Design review of the part built by this model. Coordinates are the model's own, in mm. A direction names the side the tool comes from. Round coordinates to 2 decimals unless told otherwise and drop trailing zeros. Write each loop counter-clockwise with the first axis right and the second up, starting at its lowest first coordinate (ties: lowest second). Pieces come first, ordered by that corner, then holes. Notation, with made-up numbers: (85, -32.75) -> (102, -32.75) arc R23 ccw to (102, -5.75) -> close; hole circle Ø2 at (16.25, 33). An arc over 180 degrees is marked (long way). Write item = value, one per line. Start each with the question number.
Item 1: Add section C-C, the plane x = 0. State the section outline as (y, z) points (3 decimals), then the cut area to 3 significant figures.
Item 2: Machinability: for faces 1 (the flat face through (6, 0, 0)), 2 (the flat face through (0, 6, -10.833)), 3 (the cylindrical face through (9.067, -14.592, 2.855)), 4 (the flat face through (-6, 0, 0)), 5 (the cylindrical face through (6.948, -6.721, 2.188)), which of the approach directions +Z, -Z, +X, -X, +Y, -Y give a long, thin tool a straight path to every point of the face, cutting with its end or side? Answer none if there is none.
Item 3: Add section B-B, the plane x = -8. State the section outline as (y, z) points (3 decimals).
Item 4: Mouldability with a two-part tool opening along Y and no side actions: class faces 6 (the flat face through (3.203, 6, 0)), 7 (the flat face through (0, -21.031, 0)), 8 (the flat face through (5, -8.331, -6)) as released by +Y, released by -Y, zero draft, split by the parting line, or undercut.
Item 5: To check wall thickness, follow L1, parallel to Y at x = -1.5, z = 8.25; L2, parallel to Y at x = -5, z = -7; L3, parallel to X at y = 10.5, z = -2.25. State the ranges of each line that lie inside material, in increasing order.
Item 6: Add section D-D, the plane y = -16. State the section outline as (x, z) points, then the cut area to 3 significant figures.
Item 7: For pin 1 Ø10 at (y, z) = (-1, 7) entering from -X; pin 2 Ø2.5 at (x, z) = (6.5, 4.5) entering from +Y; pin 3 Ø2 at (y, z) = (-5.5, 8) entering from +X; pin 4 Ø1.5 at (y, z) = (-2, -0.5) entering from -X, all flat-tipped, find the tip position at first contact; note any pin that passes through.
Item 8: Add section A-A, the plane z = 0. State the section outline as (x, y) points (3 decimals), then the cut area to 3 significant figures.
from build123d import *

# Parameters (mm, degrees)
F0_R     = 11.130797
F1_DEPTH = 3.175
F2_W     = 6.405964
F2_H     = 21.666086
F3_DEPTH = 12.7
F4_R     = 9.48328
F5_DEPTH = 5.1562
F6_R     = 7.284162
F7_DEPTH = 8.3312
F8_R     = 9.506324
F9_DEPTH = 12.7


with BuildPart() as f1:
    # F0 (on Front) → F1 (new body)
    with BuildSketch(Plane.XZ):
        Circle(F0_R)
    extrude(amount=F1_DEPTH)

    # F2 (on Front) → F3 (join)
    with BuildSketch(Plane.XZ):
        Rectangle(F2_W, F2_H)
    extrude(amount=-F3_DEPTH)

    # F4 (on Front) → F5 (join)
    with BuildSketch(Plane.XZ):
        Circle(F4_R)
    extrude(amount=F5_DEPTH)

    # F6 (on Front) → F7 (join)
    with BuildSketch(Plane.XZ):
        Circle(F6_R)
    extrude(amount=F7_DEPTH)

    # F8 (on face) → F9 (join)
    with BuildSketch(Plane.XZ.offset(8.3312)):
        Circle(F8_R)
    extrude(amount=F9_DEPTH)


solid = f1.part
Result set:
q1.outline = (-21.031, -9.506) -> (-8.331, -9.506) -> (-8.331, -7.284) -> (-5.156, -7.284) -> (-5.156, -9.483) -> (-3.175, -9.483) -> (-3.175, -11.131) -> (0, -11.131) -> (0, -10.833) -> (12.7, -10.833) -> (12.7, 10.833) -> (0, 10.833) -> (0, 11.131) -> (-3.175, 11.131) -> (-3.175, 9.483) -> (-5.156, 9.483) -> (-5.156, 7.284) -> (-8.331, 7.284) -> (-8.331, 9.506) -> (-21.031, 9.506) -> close
q1.area = 671 mm²
q2.face_1 = +Z, -Z, +X, +Y
q2.face_2 = -Z, +X, -X, +Y
q2.face_3 = -Y
q2.face_4 = +Z, -Z, -X, +Y
q2.face_5 = none
q3.outline = (-21.031, -5.135) -> (-8.331, -5.135) -> (-8.331, 5.135) -> (-21.031, 5.135) -> close; (-5.156, -5.092) -> (-3.175, -5.092) -> (-3.175, -7.739) -> (0, -7.739) -> (0, 7.739) -> (-3.175, 7.739) -> (-3.175, 5.092) -> (-5.156, 5.092) -> close
q4.face_6 = zero draft
q4.face_7 = released by -Y
q4.face_8 = undercut
q5.L1 = -21.03 to -8.33, -5.16 to 12.7
q5.L2 = -21.03 to -8.33, -5.16 to 0
q5.L3 = -3.2 to 3.2
q6.outline = circle Ø19.01 at (0, 0)
q6.area = 284 mm²
q7.pin_1 = -10.95
q7.pin_2 = 0
q7.pin_3 = 6.33
q7.pin_4 = -11.13
q8.outline = (-11.131, -3.175) -> (-9.483, -3.175) -> (-9.483, -5.156) -> (-7.284, -5.156) -> (-7.284, -8.331) -> (-9.506, -8.331) -> (-9.506, -21.031) -> (9.506, -21.031) -> (9.506, -8.331) -> (7.284, -8.331) -> (7.284, -5.156) -> (9.483, -5.156) -> (9.483, -3.175) -> (11.131, -3.175) -> (11.131, 0) -> (3.203, 0) -> (3.203, 12.7) -> (-3.203, 12.7) -> (-3.203, 0) -> (-11.131, 0) -> close
q8.area = 477 mm²
